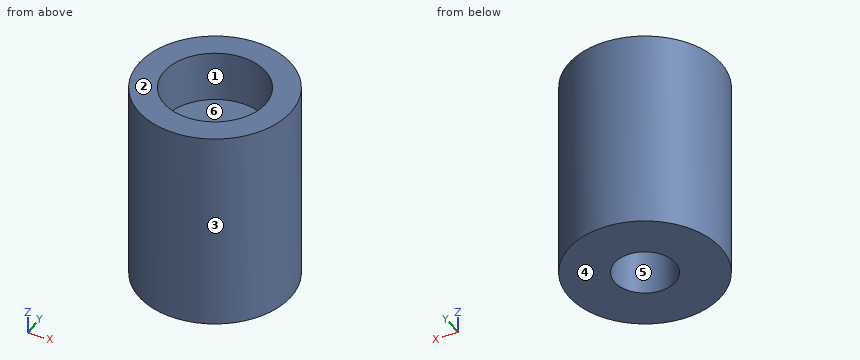
from build123d import *

# Parameters (mm, degrees)
SKETCH1_R           = 3
SKETCH1_R_2         = 2
SKETCH1_R_3         = 1.2
BOSS_EXTRUDE1_DEPTH = 8
CUT_EXTRUDE1_START  = 8
SKETCH1_3_R         = 2
SKETCH1_3_R_2       = 1.2
CUT_EXTRUDE1_DEPTH  = 2
SKETCH1_4_R         = 1.2
CUT_EXTRUDE2_DEPTH  = 5


with BuildPart() as part:
    # Sketch1 → Boss-Extrude1 (new body)
    # profile 1 of 3: a face of its own
    with BuildSketch(Plane(origin=(0, 0, 0), x_dir=(0, 1, 0), z_dir=(0, 0, 1))):
        with Locations(Location((0, 0, 0), (0, 0, 270))):
            Circle(SKETCH1_R)
        Circle(SKETCH1_R_2, mode=Mode.SUBTRACT)
    # profile 2 of 3: a face of its own
    with BuildSketch(Plane(origin=(0, 0, 0), x_dir=(0, 1, 0), z_dir=(0, 0, 1))):
        Circle(SKETCH1_R_2)
        Circle(SKETCH1_R_3, mode=Mode.SUBTRACT)
    # profile 3 of 3: a face of its own
    with BuildSketch(Plane(origin=(0, 0, 0), x_dir=(0, 1, 0), z_dir=(0, 0, 1))):
        Circle(SKETCH1_R_3)
    extrude(amount=BOSS_EXTRUDE1_DEPTH)

    # Sketch1<3> → Cut-Extrude1 (cut)
    # profile 1 of 2: a face of its own
    with BuildSketch(Plane(origin=(0, 0, 0), x_dir=(0, 1, 0), z_dir=(0, 0, 1)).offset(CUT_EXTRUDE1_START)):
        with Locations(Location((0, 0, 0), (0, 0, 270))):
            Circle(SKETCH1_3_R)
        Circle(SKETCH1_3_R_2, mode=Mode.SUBTRACT)
    # profile 2 of 2: a face of its own
    with BuildSketch(Plane(origin=(0, 0, 0), x_dir=(0, 1, 0), z_dir=(0, 0, 1)).offset(CUT_EXTRUDE1_START)):
        Circle(SKETCH1_3_R_2)
    extrude(amount=-CUT_EXTRUDE1_DEPTH, mode=Mode.SUBTRACT)

    # Sketch1<4> → Cut-Extrude2 (cut)
    with BuildSketch(Plane(origin=(0, 0, 0), x_dir=(0, 1, 0), z_dir=(0, 0, 1))):
        with Locations(Location((0, 0, 0), (0, 0, 270))):
            Circle(SKETCH1_4_R)
    extrude(amount=CUT_EXTRUDE2_DEPTH, mode=Mode.SUBTRACT)


solid = part.part
Part model, mm, in its own coordinate system. Face numbers are marked on the shaded views. A direction names the side the tool comes from. Coordinates: 2 decimals unless noted, no trailing zeros. Order: outer loops, then holes, each group sorted by start corner. A loop starts at its lowest first (then second) coordinate and runs counter-clockwise, first axis right, second up.
(1) Slice it at C-C, the plane z = 5.75. Write the cut outline in (x, y), and give its area (3 significant figures).
Check sheet entries:
outline: circle Ø6 at (0, 0)
area: 28.3 mm2
(2) Slice it at D-D, the plane z = 2.25. Write the cut outline in (x, y).
Check sheet entries:
outline: circle Ø6 at (0, 0); hole circle Ø2.4 at (0, 0)
(3) Pin check, flat tips, straight feed: pin 1 Ø2 at (y, z) = (-2, 3) entering from -X; pin 2 Ø3 at (x, y) = (0, 0) entering from +Z. Stop position of each tip, or through.
Check sheet entries:
pin 1: stops at x = -2.83
pin 2: stops at z = 6
(4) Tool access for the marked faces 1 and 2: list every direction of +Z, -Z, +X, -X, +Y, -Y with a clear straight run to the whole face (end or side of a thin tool).
Check sheet entries:
face 1: +Z
face 2: +Z, +X, -X, +Y, -Y
(5) Pull direction X, two halves, no side cores. Call the marked faces 3, 4, 5 and 6: pulls with the +X half, pulls with the -X half, needs draft (parallel to the pull), parting line crosses it, or undercut.
Check sheet entries:
face 3: parting line crosses it
face 4: needs draft
face 5: undercut
face 6: undercut
(6) Probe L1, parallel to Y at x = 0, z = 1.65; L2, parallel to Y at x = 0, z = 6.7; L3, parallel to Z at x = 1.3, y = -1. List the from-to ranges inside material, lowest first.
Check sheet entries:
L1: y = -3 to -1.2, 1.2 to 3
L2: y = -3 to -2, 2 to 3
L3: z = 0 to 6
(7) Slice it at A-A, the plane x = 0. Write the cut outline in (y, z).
Check sheet entries:
outline: (-3, 0) - (-1.2, 0) - (-1.2, 5) - (1.2, 5) - (1.2, 0) - (3, 0) - (3, 8) - (2, 8) - (2, 6) - (-2, 6) - (-2, 8) - (-3, 8) - close
